Check sheet for the modelled part. Datum: model origin and axes. Units: mm. A direction names the side the tool comes from. Round coordinates to 2 decimals unless told otherwise and drop trailing zeros. Write each loop counter-clockwise with the first axis right and the second up, starting at its lowest first coordinate (ties: lowest second). Pieces come first, ordered by that corner, then holes. Notation, with made-up numbers: (42, 0.5) -> (53, 0.5) arc R12 ccw to (53, 21.5) -> close; hole circle Ø4 at (57, -35.75). An arc over 180 degrees is marked (long way). One line per item, written item: value.
from build123d import *

# Parameters (mm, degrees)
F1_DEPTH = 66
F2_R     = 2
F3_DEPTH = 25
F4_R     = 1.5
F5_DEPTH = 25
F6_R     = 1
F7_DEPTH = 25


# Not quite as in the source:
# - a feature names something its author has since deleted; it is built from what else it names


with BuildPart() as f1:
    # F0 (on Top) → F1 (new body)
    with BuildSketch(Plane.XY):
        with BuildLine():
            Line((-66.75, -33), (-66.75, 33))
            Line((-66.75, 33), (-68.25, 33))
            Line((-68.25, 33), (-68.25, -33))
            ThreePointArc((-68.25, -33), (-66.7855339059, -36.5355339059), (-63.25, -38))
            Line((-63.25, -38), (48.75, -38))
            ThreePointArc((48.75, -38), (52.2855339059, -36.5355339059), (53.75, -33))
            Line((53.75, -33), (53.75, 33))
            ThreePointArc((53.75, 33), (52.2855339059, 36.5355339059), (48.75, 38))
            Line((48.75, 38), (-48.75, 38))
            ThreePointArc((-48.75, 38), (-52.2855339059, 36.5355339059), (-53.75, 33))
            Line((-53.75, 33), (-53.75, 0))
            Line((-53.75, 0), (-52.25, 0))
            Line((-52.25, 0), (-52.25, 33))
            ThreePointArc((-52.25, 33), (-51.2248737342, 35.4748737342), (-48.75, 36.5))
            Line((-48.75, 36.5), (48.75, 36.5))
            ThreePointArc((48.75, 36.5), (51.2248737342, 35.4748737342), (52.25, 33))
            Line((52.25, 33), (52.25, -33))
            ThreePointArc((52.25, -33), (51.2248737342, -35.4748737342), (48.75, -36.5))
            Line((48.75, -36.5), (-63.25, -36.5))
            ThreePointArc((-63.25, -36.5), (-65.7248737342, -35.4748737342), (-66.75, -33))
        make_face()
    extrude(amount=F1_DEPTH)

    # F2 (on face) → F3 (cut)
    with BuildSketch(Plane.XZ.offset(38)):
        with BuildLine():
            Line((20.75, 52), (-23.25, 52))
            ThreePointArc((-23.25, 52), (-25.3713203436, 51.1213203436), (-26.25, 49))
            Line((-26.25, 49), (-26.25, 17))
            ThreePointArc((-26.25, 17), (-25.3713203436, 14.8786796564), (-23.25, 14))
            Line((-23.25, 14), (20.75, 14))
            ThreePointArc((20.75, 14), (22.8713203436, 14.8786796564), (23.75, 17))
            Line((23.75, 17), (23.75, 49))
            ThreePointArc((23.75, 49), (22.8713203436, 51.1213203436), (20.75, 52))
        make_face()
        with Locations((-26.25, 58)):
            Circle(F2_R)
        with Locations((23.75, 58)):
            Circle(F2_R)
        with Locations((23.75, 8)):
            Circle(F2_R)
        with Locations((-26.25, 8)):
            Circle(F2_R)
        with BuildLine():
            ThreePointArc((-8.75, 8.5), (-8.3106601718, 7.4393398282), (-7.25, 7))
            Line((-7.25, 7), (4.75, 7))
            ThreePointArc((4.75, 7), (5.8106601718, 7.4393398282), (6.25, 8.5))
            ThreePointArc((6.25, 8.5), (5.8106601718, 9.5606601718), (4.75, 10))
            Line((4.75, 10), (-7.25, 10))
            ThreePointArc((-7.25, 10), (-8.3106601718, 9.5606601718), (-8.75, 8.5))
        make_face()
        with Locations((-20.25, 8)):
            Circle(F2_R)
        with Locations((-20.25, 58)):
            Circle(F2_R)
        with Locations((17.75, 58)):
            Circle(F2_R)
        with Locations((14.75, 8)):
            Circle(F2_R)
    extrude(amount=-F3_DEPTH, mode=Mode.SUBTRACT)

    # F4 (on face) → F5 (cut)
    with BuildSketch(Plane(origin=(0, 38, 0), x_dir=(-1, 0, 0), z_dir=(0, 1, 0))):
        with Locations((-40, 58)):
            Circle(F4_R)
        with Locations((-40, 8)):
            Circle(F4_R)
        with Locations((40, 8)):
            Circle(F4_R)
        with Locations((40, 58)):
            Circle(F4_R)
        with Locations((40, 16.5)):
            Circle(F4_R)
        with Locations((40, 49.5)):
            Circle(F4_R)
    extrude(amount=-F5_DEPTH, mode=Mode.SUBTRACT)

    # F6 (on face) → F7 (cut)
    with BuildSketch(Plane.YZ.offset(53.75)):
        with BuildLine():
            Line((-17, 58), (-21, 58))
            ThreePointArc((-21, 58), (-23.1213203436, 57.1213203436), (-24, 55))
            Line((-24, 55), (-24, 11))
            ThreePointArc((-24, 11), (-23.1213203436, 8.8786796564), (-21, 8))
            Line((-21, 8), (-17, 8))
            ThreePointArc((-17, 8), (-14.8786796564, 8.8786796564), (-14, 11))
            Line((-14, 11), (-14, 55))
            ThreePointArc((-14, 55), (-14.8786796564, 57.1213203436), (-17, 58))
        make_face()
        with BuildLine():
            Line((24, 58), (-5, 58))
            ThreePointArc((-5, 58), (-7.1213203436, 57.1213203436), (-8, 55))
            Line((-8, 55), (-8, 11))
            ThreePointArc((-8, 11), (-7.1213203436, 8.8786796564), (-5, 8))
            Line((-5, 8), (24, 8))
            ThreePointArc((24, 8), (26.1213203436, 8.8786796564), (27, 11))
            Line((27, 11), (27, 55))
            ThreePointArc((27, 55), (26.1213203436, 57.1213203436), (24, 58))
        make_face()
        with Locations((-19, 61)):
            Circle(F6_R)
        with Locations((9.5, 61)):
            Circle(F6_R)
        with Locations((9.5, 5)):
            Circle(F6_R)
        with Locations((-19, 5)):
            Circle(F6_R)
    extrude(amount=-F7_DEPTH, mode=Mode.SUBTRACT)


solid = f1.part
Item 1: Sectioned sample at C-C (y = 12.5). Enter the section's corners in (x, z).
Result set:
outline: (-68.25, 0) -> (-66.75, 0) -> (-66.75, 66) -> (-68.25, 66) -> close; (-53.75, 0) -> (-52.25, 0) -> (-52.25, 66) -> (-53.75, 66) -> close; (52.25, 0) -> (53.75, 0) -> (53.75, 8) -> (52.25, 8) -> close; (52.25, 58) -> (53.75, 58) -> (53.75, 66) -> (52.25, 66) -> close
Item 2: Sectioned sample at A-A (x = -40). Enter the section's corners in (y, z).
Result set:
outline: (-38, 0) -> (-36.5, 0) -> (-36.5, 66) -> (-38, 66) -> close; (36.5, 0) -> (38, 0) -> (38, 6.5) -> (36.5, 6.5) -> close; (36.5, 9.5) -> (38, 9.5) -> (38, 15) -> (36.5, 15) -> close; (36.5, 18) -> (38, 18) -> (38, 48) -> (36.5, 48) -> close; (36.5, 51) -> (38, 51) -> (38, 56.5) -> (36.5, 56.5) -> close; (36.5, 59.5) -> (38, 59.5) -> (38, 66) -> (36.5, 66) -> close
Item 3: Material ranges on line 1 along X through (y, z) = (9.5, 3.5); line 2 along Z through (x, y) = (-40, 37.35); line 3 along Z through (x, y) = (14.75, -36.95), recorded low to high.
Result set:
line 1: -68.25 to -66.75, -53.75 to -52.25, 52.25 to 53.75
line 2: 0 to 6.5, 9.5 to 15, 18 to 48, 51 to 56.5, 59.5 to 66
line 3: 0 to 6, 10 to 14, 52 to 66
Item 4: Sectioned sample at B-B (z = 34). State how many separate pieces and enclosed holes the cut face has, then the cut area to 3 significant figures.
Result set:
separate pieces: 4
enclosed holes: 0
area: 459 mm^2
Item 5: Release check for a two-part mould opening along Y. For faces 1 (the flat face through (-52.25, 16, 33)), 2 (the cylindrical face through (52.32, 36.5, 32.54)), 3 (the cylindrical face through (13.276, -37.26, 9.352)) record: pulls with the +Y half, pulls with the -Y half, needs draft (parallel to the pull), parting line crosses it, or undercut.
Result set:
face 1: undercut
face 2: pulls with the +Y half
face 3: needs draft
Item 6: Tool access check on faces 4 (the cylindrical face through (22.89, -37.26, 51.1)), 5 (the cylindrical face through (53.01, -7.1, 57.14)), 6 (the flat face through (52.25, 30, 33)). Record the directions out of +Z, -Z, +X, -X, +Y, -Y that give a thin tool (end or side, any length) a straight path to the whole face; none if there is none.
Result set:
face 4: -Y
face 5: +X
face 6: +Z, -Z
Item 7: Sectioned sample at D-D (x = 40). Enter the section's corners in (y, z).
Result set:
outline: (-38, 0) -> (-36.5, 0) -> (-36.5, 66) -> (-38, 66) -> close; (36.5, 0) -> (38, 0) -> (38, 6.5) -> (36.5, 6.5) -> close; (36.5, 9.5) -> (38, 9.5) -> (38, 56.5) -> (36.5, 56.5) -> close; (36.5, 59.5) -> (38, 59.5) -> (38, 66) -> (36.5, 66) -> close
Item 8: Depth check by flat-ended pin: pin 1 (1.6 mm diameter, centred on x = 52.5, z = 29, fed in from -Y); pin 2 (1.5 mm diameter, centred on y = -21, z = 56, fed in from +X); pin 3 (3 mm diameter, centred on x = 17.75, z = 58, fed in from -Y). Enter the tip coordinate at first touch or a pass-through.
Result set:
pin 1: y = -37.04
pin 2: x = -66.75
pin 3: y = 36.5
